Autodesk Inventor part; units mm, degrees
ref_plane "Work Plane1" through (0, 12.5, 0) normal (0, 1, 0) x (-1, 0, 0)
ref_plane "YZ Plane" through (0, 0, 0) normal (1, 0, 0) x (0, 1, 0)
ref_plane "XY Plane" through (0, 0, 0) normal (0, 0, 1) x (1, 0, 0)
sketch "Sketch1" plane through (0, 0, 0) normal (0, 1, 0) x (-1, 0, 0)
  circle A0 centre (0, 0) radius 9.7
  dimension "d0" = 19.4
ref_plane "Work Plane1" through (0, 12.5, 0) normal (0, 1, 0) x (-1, 0, 0)
sketch "Sketch2" plane through (0, 12.5, 0) normal (0, 1, 0) x (-1, 0, 0)
  circle A0 centre (0, 0) radius 12.5
  dimension "d2" = 25
loft "Loft1" add profiles "Sketch1", "Sketch2"
sketch "Sketch5" plane through (0, 12.5, 0) normal (0, 1, 0) x (1, 0, 0)
  circle A0 centre (0, 0) radius 12.5
  dimension "d9" = 25
extrude "Extrusion1" add sketch "Sketch5" along normal blind 11.5
sketch "Sketch6" plane through (0, 24, 0) normal (0, 1, 0) x (1, 0, 0)
  circle A0 centre (0, 0) radius 9.65
  dimension "d12" = 19.3
extrude "Extrusion2" add sketch "Sketch6" along normal blind 13.55
sketch "Sketch7" plane through (0, 37.55, 0) normal (0, 1, 0) x (1, 0, 0)
  line L0 (-6.3788, -11.1172) -> (-12.8171, -0.0344)
  line L1 (-12.8171, -0.0344) -> (-6.4384, 11.0828)
  line L2 (-6.4384, 11.0828) -> (6.3788, 11.1172)
  line L3 (6.3788, 11.1172) -> (12.8171, 0.0344)
  line L4 (12.8171, 0.0344) -> (6.4384, -11.0828)
  line L5 (6.4384, -11.0828) -> (-6.3788, -11.1172)
  point P0 (0, 0)
  point P1 (0, 0)
  dimension "d15" = 22.2
extrude "Extrusion3" add sketch "Sketch7" along normal blind 19.15
sketch "Sketch8" plane through (0, 56.7, 0) normal (0, 1, 0) x (1, 0, 0)
  circle A0 centre (0, 0) radius 9.05
  dimension "d18" = 18.1
extrude "Extrusion4" add sketch "Sketch8" along normal blind 11
sketch "Sketch9" plane through (0, 67.7, 0) normal (0, 1, 0) x (1, 0, 0)
  circle A0 centre (0, 0) radius 6.35
  dimension "d21" = 12.7
extrude "Extrusion5" add sketch "Sketch9" along normal blind 14
sketch "Sketch10" plane through (0, 81.7, 0) normal (0, 1, 0) x (1, 0, 0)
  circle A0 centre (0, 0) radius 6.35
  dimension "d26" = 12.7
extrude "Extrusion6" add sketch "Sketch10" along normal blind 46
thread "Thread2"
chamfer "Chamfer1" distance 0.5 angle 45 1 edges at (-12.5, 24, 0)
properties part number "Soporte Bailarina" material "Steel, Alloy"
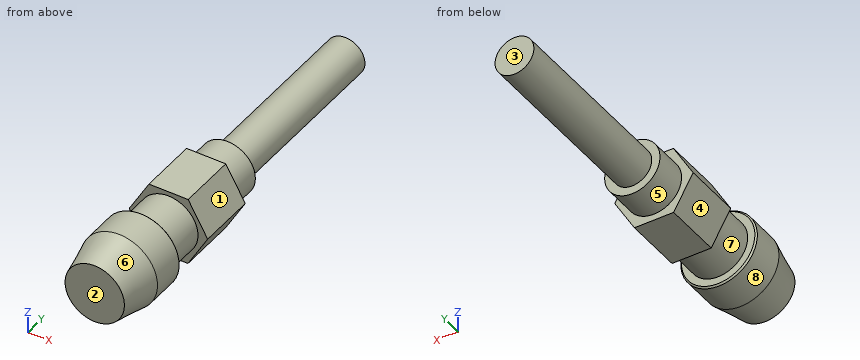
Design review of the part built by this model. Coordinates are the model's own, in mm. Face numbers are marked on the shaded views. A direction names the side the tool comes from. Give positions to 0.01 mm unless a question says otherwise; leave off trailing zeros. Write each loop counter-clockwise with the first axis right and the second up, starting at its lowest first coordinate (ties: lowest second). Pieces come first, ordered by that corner, then holes. Notation, with made-up numbers: (85.5, -24) - (121.5, -24) arc R19 ccw to (121.5, -9) - close; hole circle Ø9 at (73.25, 20.25). An arc over 180 degrees is marked (long way). Return JSON: item names as keys, results as strings. Group by question number.
(1) To check wall thickness, follow probe 1 along Y at (x, z) = (7.25, -4.25); probe 2 along X at (y, z) = (49, 5.5); probe 3 along X at (y, z) = (11.5, -7.5). State the ranges of each line that lie inside material, in increasing order.
(2) We need section A-A, the plane y = 51.5. Give the boundary of the cut face in (x, z).
(3) Insertion check: pin 1 (1 mm diameter, centred on x = -9.5, z = 10, fed in from -Y); pin 2 (2 mm diameter, centred on y = 81.5, z = -1.5, fed in from -X); pin 3 (12 mm diameter, centred on y = 105, z = -4, fed in from +X); pin 4 (12 mm diameter, centred on x = -8, y = 20.5, fed in from -Z). Each pin has a flat end and moves straight along its axis. Give the tip position at first contact, or say it passes through.
(4) We need section D-D, the plane y = 102. Give the boundary of the cut face in (x, z).
(5) We need section B-B, the plane x = 0. Give the boundary of the cut face in (y, z), then the cut area to 3 significant figures.
(6) We need section C-C, the plane y = 16. Give the boundary of the cut face in (x, z), then the cut area to 3 significant figures.
(7) Machinability: for the marked faces 1, 2, 3, 4 and 5, which of the approach directions +Z, -Z, +X, -X, +Y, -Y give a long, thin tool a straight path to every point of the face, cutting with its end or side? Answer none if there is none.
(8) Mouldability with a two-part tool opening along Y and no side actions: class the marked faces 6, 7 and 8 as +Y half, -Y half, draft (parallel to the pull), parting line (faces both ways), or undercut.
Reported:
{
 "1": {"probe 1": "y = 0 to 67.7", "probe 2": "x = -9.64 to 9.64", "probe 3": "x = -9.72 to 9.72"},
 "2": {"outline": "(-12.82, 0.03) - (-6.44, -11.08) - (6.38, -11.12) - (12.82, -0.03) - (6.44, 11.08) - (-6.38, 11.12) - close"},
 "3": {"pin 1": "passes through", "pin 2": "stops at x = -6.33", "pin 3": "stops at x = 6.35", "pin 4": "stops at z = -12.34"},
 "4": {"outline": "circle Ø12.7 at (0, 0)"},
 "5": {"outline": "(0, -9.7) - (12.5, -12.5) - (23.5, -12.5) - (24, -12) - (24, -9.65) - (37.55, -9.65) - (37.55, -11.1) - (56.7, -11.1) - (56.7, -9.05) - (67.7, -9.05) - (67.7, -6.35) - (127.7, -6.35) - (127.7, 6.35) - (67.7, 6.35) - (67.7, 9.05) - (56.7, 9.05) - (56.7, 11.1) - (37.55, 11.1) - (37.55, 9.65) - (24, 9.65) - (24, 12) - (23.5, 12.5) - (12.5, 12.5) - (0, 9.7) - close", "area": "2,210 mm2"},
 "6": {"outline": "circle Ø25 at (0, 0)", "area": "491 mm2"},
 "7": {"face 1": "+Z, +X, +Y", "face 2": "+Z, -Z, +X, -X, -Y", "face 3": "+Z, -Z, +X, -X, +Y", "face 4": "-Z, -X, +Y", "face 5": "+Y"},
 "8": {"face 6": "-Y half", "face 7": "undercut", "face 8": "draft"}
}
